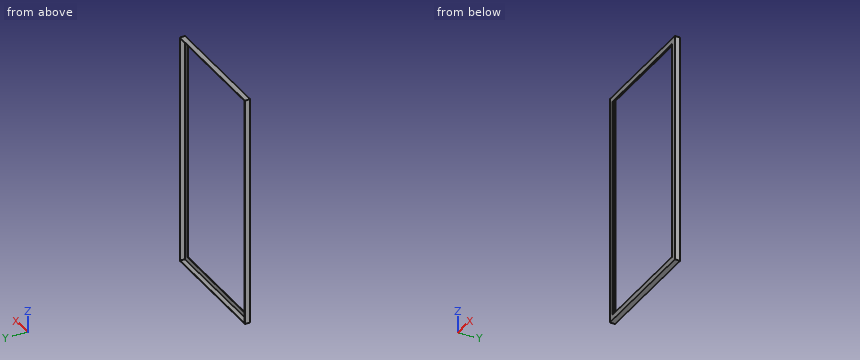
Autodesk Inventor part; units mm, degrees
ref_plane "YZ Plane" through (0, 0, 0) normal (1, 0, 0) x (0, 1, 0)
ref_plane "XZ Plane" through (0, 0, 0) normal (0, 1, 0) x (-1, 0, 0)
ref_plane "XY Plane" through (0, 0, 0) normal (0, 0, 1) x (1, 0, 0)
sketch "Sketch1" plane through (0, 0, 0) normal (0, 1, 0) x (-1, 0, 0)
  line L0 (-406, 0) -> (406, 0) construction
  line L1 (0, -773.5) -> (0, 773.5) construction
  line L2 (290, 552.5) -> (-290, 552.5)
  line L3 (-290, 552.5) -> (-290, -552.5)
  line L4 (-290, -552.5) -> (290, -552.5)
  line L5 (290, -552.5) -> (290, 552.5)
  line L6 (264.6, -527.1) -> (-264.6, -527.1)
  line L7 (-264.6, -527.1) -> (-264.6, 527.1)
  line L8 (-264.6, 527.1) -> (264.6, 527.1)
  line L9 (264.6, 527.1) -> (264.6, -527.1)
  point P0 (0, 0)
  dimension "d0" = 580
  dimension "d1" = 1105
  dimension "d8" = 25.4
  dimension "d9" = 25.4
extrude "Base thickness" add sketch "Sketch1" along normal blind 3
sketch "Sketch3" plane through (0, 3, 0) normal (0, 1, 0) x (1, 0, 0)
  line L0 (-290, 552.5) -> (-290, -552.5)
  line L1 (-290, -552.5) -> (290, -552.5)
  line L2 (290, -552.5) -> (290, 552.5)
  line L3 (290, 552.5) -> (-290, 552.5)
  line L4 (-290, 552.5) -> (-290, -552.5)
  line L5 (-287, 549.5) -> (287, 549.5)
  line L6 (287, 549.5) -> (287, -549.5)
  line L7 (287, -549.5) -> (-287, -549.5)
  line L8 (-287, -549.5) -> (-287, 549.5)
  line L9 (0, 773.5) -> (0, -773.5) construction
  line L10 (406, 0) -> (-406, 0) construction
  point P0 (0, 0)
  dimension "d14" = 3
  dimension "d15" = 3
extrude "Wall height" add sketch "Sketch3" along normal blind 22.4
equation "\"d8\" = angleSectionSize"
equation "\"d9\" = angleSectionSize"
equation "\"d12\" = wallThickness"
equation "\"d14\" = wallThickness"
equation "\"d15\" = wallThickness"
equation "\"d16\" = angleSectionSize - wallThickness"
equation "\"wallThickness\" = 3"
equation "\"angleSectionSize\" = 25.4"
properties part number "frame" material "Steel, Mild"
Could you check a few things on this model? Use its own coordinates, in mm. Give positions to 0.01 mm unless a question says otherwise; leave off trailing zeros. Order: outer loops, then holes, each group sorted by start corner. A loop starts at its lowest first (then second) coordinate and runs counter-clockwise, first axis right, second up. Notation, with made-up numbers: (9.25, 74) - (34.25, 74) arc R22 cw to (34.25, 107) - close; hole circle Ø5 at (35.25, 77). An arc over 180 degrees is marked (long way). One line per question, with ' | ' between items. Start each with the question number.
Item 1: I need wall thicknesses on probe 1 along Z at (x, y) = (80, 19.5); probe 2 along X at (y, z) = (3.25, -36.5); probe 3 along Z at (x, y) = (194, 2). Which ranges of each line are inside material? Lowest first, please. Write a range as [from, to].
Item 2: I want a section at B-B on y = 13.75. Write out the boundary of the cut face in (x, z), then the cut area to 3 significant figures.
Item 3: I want a section at C-C on x = -114. Write out the boundary of the cut face in (y, z), then the cut area to 3 significant figures.
Item 4: I want a section at A-A on z = 22. Write out the boundary of the cut face in (x, y).
Verdict:
1) probe 1: [-552.5, -549.5], [549.5, 552.5] | probe 2: [-290, -287], [287, 290] | probe 3: [-552.5, -527.1], [527.1, 552.5]
2) outline: (-290, -552.5) - (290, -552.5) - (290, 552.5) - (-290, 552.5) - close; hole (-287, -549.5) - (287, -549.5) - (287, 549.5) - (-287, 549.5) - close | area: 10,100 mm^2
3) outline: (0, -552.5) - (25.4, -552.5) - (25.4, -549.5) - (3, -549.5) - (3, -527.1) - (0, -527.1) - close; (0, 527.1) - (3, 527.1) - (3, 549.5) - (25.4, 549.5) - (25.4, 552.5) - (0, 552.5) - close | area: 287 mm^2
4) outline: (-290, 0) - (-264.6, 0) - (-264.6, 3) - (-287, 3) - (-287, 25.4) - (-290, 25.4) - close; (264.6, 0) - (290, 0) - (290, 25.4) - (287, 25.4) - (287, 3) - (264.6, 3) - close
